from build123d import *

# Parameters (mm, degrees)
F2_DEPTH = 92.5154741853
F0_DEPTH = 97.1629172564


with BuildPart() as f2:
    # F1 (on Top) → F2 (new body)
    with BuildSketch(Plane.XY):
        with BuildLine():
            ThreePointArc((44.535878433, -33.2482290868), (69.3702098075, -24.249252625), (79.8439550455, 0))
            ThreePointArc((79.8439550455, 0), (75.8514189323, 15.8123037264), (64.8309496766, 27.8338906072))
            ThreePointArc((64.8309496766, 27.8338906072), (52.8981608399, 6.706864812), (34.3638503598, -8.9527010632))
            ThreePointArc((34.3638503598, -8.9527010632), (41.2778387441, -20.3351305507), (44.535878433, -33.2482290868))
        make_face()
        with BuildLine():
            ThreePointArc((34.3638503598, -8.9527010632), (52.8981608399, 6.706864812), (64.8309496766, 27.8338906072))
            ThreePointArc((64.8309496766, 27.8338906072), (32.9810423523, 30.4255919297), (13.6068053003, 5.0135386682))
            ThreePointArc((13.6068053003, 5.0135386682), (24.9811912081, -0.4894991276), (34.3638503598, -8.9527010632))
        make_face()
        with BuildLine():
            ThreePointArc((13.6068053003, 5.0135386682), (32.9810423523, 30.4255919297), (64.8309496766, 27.8338906072))
            ThreePointArc((64.8309496766, 27.8338906072), (67.7145282445, 39.013298427), (68.6848598779, 50.5177602172))
            ThreePointArc((68.6848598779, 50.5177602172), (-21.7831497836, 115.6568756699), (-54.8679687803, 9.2005001631))
            ThreePointArc((-54.8679687803, 9.2005001631), (-27.6196679815, 25.597862276), (-1.7527016438, 7.0980397588))
            ThreePointArc((-1.7527016438, 7.0980397588), (6.0179921547, 6.7258769298), (13.6068053003, 5.0135386682))
        make_face()
        with BuildLine():
            ThreePointArc((44.7496727734, -37.6172959805), (44.6961922309, -35.4301486637), (44.535878433, -33.2482290868))
            ThreePointArc((44.535878433, -33.2482290868), (28.6822600259, -28.119398588), (17.2965115244, -15.9535919997))
            ThreePointArc((17.2965115244, -15.9535919997), (6.8156269651, -17.8281043653), (-3.8290350442, -18.0602863216))
            ThreePointArc((-3.8290350442, -18.0602863216), (-21.6809587163, -31.4155799712), (-43.73192107, -28.1277073248))
            ThreePointArc((-43.73192107, -28.1277073248), (-4.7720045941, -82.1118033435), (44.7496727734, -37.6172959805))
        make_face()
        with BuildLine():
            ThreePointArc((17.2965115244, -15.9535919997), (28.6822600259, -28.119398588), (44.535878433, -33.2482290868))
            ThreePointArc((44.535878433, -33.2482290868), (41.2778387441, -20.3351305507), (34.3638503598, -8.9527010632))
            ThreePointArc((34.3638503598, -8.9527010632), (26.0662879209, -13.0287472437), (17.2965115244, -15.9535919997))
        make_face()
        with BuildLine():
            ThreePointArc((-34.3638503598, -8.9527010632), (-19.7612727928, 2.5327390249), (-1.7527016438, 7.0980397588))
            ThreePointArc((-1.7527016438, 7.0980397588), (-27.6196679815, 25.597862276), (-54.8679687803, 9.2005001631))
            ThreePointArc((-54.8679687803, 9.2005001631), (-45.5298151265, -0.9083606845), (-34.3638503598, -8.9527010632))
        make_face()
        with BuildLine():
            ThreePointArc((-34.3638503598, -8.9527010632), (-45.5298151265, -0.9083606845), (-54.8679687803, 9.2005001631))
            ThreePointArc((-54.8679687803, 9.2005001631), (-56.5144673123, -11.6158972728), (-43.73192107, -28.1277073248))
            ThreePointArc((-43.73192107, -28.1277073248), (-40.2076807972, -17.9735789636), (-34.3638503598, -8.9527010632))
        make_face()
        with BuildLine():
            ThreePointArc((-43.73192107, -28.1277073248), (-21.6809587163, -31.4155799712), (-3.8290350442, -18.0602863216))
            ThreePointArc((-3.8290350442, -18.0602863216), (-19.6318911769, -15.3016808718), (-34.3638503598, -8.9527010632))
            ThreePointArc((-34.3638503598, -8.9527010632), (-40.2076807972, -17.9735789636), (-43.73192107, -28.1277073248))
        make_face()
    extrude(amount=F2_DEPTH)

    # F3 (on Top) → F0 (join)
    with BuildSketch(Plane.XY):
        with BuildLine():
            add(Edge.make_bspline(
                [(-34.9871255457, -10.5970427394), (-38.5202182083, -7.629362708), (-26.9744975771, 3.3374806038), (20.1910972985, 24.1151109584), (50.3086010226, -22.7421521605), (-26.7868217781, -17.4850244785), (-34.9871255457, -10.5970427394)],
                knots=[0, 0, 0, 0, 0.1481479543, 0.4463197978, 0.6561487784, 1, 1, 1, 1], degree=3))
        make_face()
    extrude(amount=F0_DEPTH)


solid = f2.part
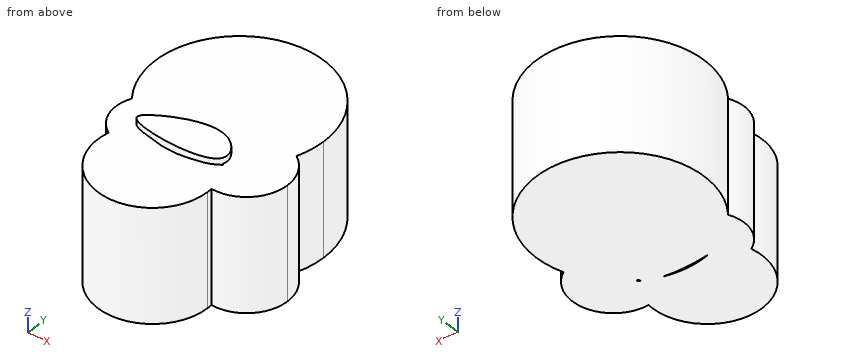
Verification items for the finished model (mm, model axes). Round coordinates to 2 decimals unless told otherwise and drop trailing zeros. Loops run counter-clockwise (first coordinate to the right, second up) from the corner with the lowest first, then second, coordinate; pieces in that order, holes last. Notation, with made-up numbers: (-30, -7) - (-26, -7) arc R24 cw to (-26, 19) - close; hole circle Ø8 at (89.25, -6.75). An arc over 180 degrees is marked (long way). Use a Markdown table: item, result. Add a question column.
1. Section check C-C, the plane x = 59. Record the boundary of the cut face in (y, z).
2. Section check B-B, the plane y = -48. Record the boundary of the cut face in (x, z), plus the area to 3 significant figures.
3. Thickness scan on probe 1 along Y at (x, z) = (1, 18); probe 2 along Z at (x, y) = (0.5, -67.5); probe 3 along X at (y, z) = (51.5, 13). Record the ranges inside material, lowest first. Write a range as [from, to].
4. Gauge pin test, flat ends, axial feed: pin 1 (1.5 mm diameter, centred on y = 35, z = 35, fed in from -X); pin 2 (2 mm diameter, centred on x = -25.5, y = -37, fed in from +Z); pin 3 (3 mm diameter, centred on y = 23, z = 65, fed in from -X); pin 4 (1.5 mm diameter, centred on x = 43.5, y = 30, fed in from -Z). Record the tip position at first contact, or that the pin passes through.
5. Section check A-A, the plane z = 6.5. Give the number of separate pieces and of enclosed holes in the cut face, plus the area to 3 significant figures.
Checks:
| question | item | result |
|---|---|---|
| 1 | outline | (-30.89, 0) - (85.68, 0) - (85.68, 92.52) - (-30.89, 92.52) - close |
| 2 | outline | (-43.53, 0) - (43.53, 0) - (43.53, 92.52) - (-43.53, 92.52) - close |
| 2 | area | 8,050 mm^2 |
| 3 | probe 1 | y = [-82.36, -18.16], [-16.99, 119.2] |
| 3 | probe 2 | z = [0, 92.52] |
| 3 | probe 3 | x = [-68.68, 68.68] |
| 4 | pin 1 | stops at x = -67.08 |
| 4 | pin 2 | stops at z = 92.52 |
| 4 | pin 3 | stops at x = -63.57 |
| 4 | pin 4 | stops at z = 0 |
| 5 | separate pieces | 1 |
| 5 | enclosed holes | 2 |
| 5 | area | 21,900 mm^2 |
